Can you work these out from the model? Positions are in its coordinate system, mm. Face numbers are marked on the shaded views. A direction names the side the tool comes from. Coordinates: 2 decimals unless noted, no trailing zeros. Loops run counter-clockwise (first coordinate to the right, second up) from the corner with the lowest first, then second, coordinate; pieces in that order, holes last. Notation, with made-up numbers: (22.25, 46.5) -> (51.25, 46.5) arc R23 ccw to (51.25, 59.5) -> close; hole circle Ø10 at (34, 81.5). An arc over 180 degrees is marked (long way). Put each result on its own line as item: value. Start each with the question number.
Item 1: If we section it at A-A on x = -40.62: Please give me the cut outline in (y, z) (3 decimals), plus the area to 3 significant figures.
Item 2: For the marked faces 1, 2 and 3, which set-ups out of +Z, -Z, +X, -X, +Y, -Y let a thin tool reach every point of the face, with its end or its side?
Item 3: We'd pull the mould along X, two halves only. Please class the marked faces 4, 5, 6 and 7: pulls with the +X half, pulls with the -X half, needs draft (parallel to the pull), parting line crosses it, or undercut.
Item 4: If we section it at D-D on x = -27: Please give me the cut outline in (y, z).
Item 5: Will these pins go through, and if not, where does the flat tip stop? P1, Ø3, axis at x = -40.5, z = 4.5, coming from the +Y side; P2, Ø4, axis at x = -40.62, z = 20.685, coming from the -Y side; P3, Ø4, axis at y = 10.5, z = 16.5, coming from the -X side; P4, Ø3.5, axis at x = -15, z = 27.5, coming from the +Y side.
Item 6: Please list where these lines run through material, in increasing order: L1, parallel to X at y = 1.5, z = 23.38 (3 decimals); L2, parallel to Z at x = -14.5, y = 3.5; L3, parallel to X at y = 7.5, z = 2.5. Write a range as from..to.
Item 7: If we section it at B-B on y = 10: Please give me the cut outline in (x, z), plus the area to 3 significant figures.
Item 8: If we section it at C-C on z = 11: Please give me the cut outline in (x, y).
```python
from build123d import *

# Parameters (mm, degrees)
BOSS_EXTRUDE1_DEPTH = 3
BOSS_EXTRUDE2_START = 3
SKETCH1_3_W         = 52.27
SKETCH1_3_H         = 26.56
BOSS_EXTRUDE2_DEPTH = 8.6
BOSS_EXTRUDE3_START = 3
SKETCH1_4_R         = 1.25
SKETCH1_4_R_2       = 5
BOSS_EXTRUDE3_DEPTH = 3.4
CUT_EXTRUDE1_REACH  = 65.526
SKETCH2_W           = 18
SKETCH2_H           = 3.5
CUT_EXTRUDE2_REACH  = 65.627
SKETCH4_W           = 12
SKETCH4_H           = 6.2
SKETCH1_5_R         = 1.25
CUT_EXTRUDE3_DEPTH  = 64.410066236


with BuildPart() as part:
    # Sketch1 → Boss-Extrude1 (new body)
    with BuildSketch(Plane(origin=(0, 0, 0), x_dir=(1, 0, 0), z_dir=(0, 1, 0))):
        with BuildLine():
            Line((-0.75, 3.25), (-51.02, 3.25))
            ThreePointArc((-51.02, 3.25), (-53.848427125, 2.078427125), (-55.02, -0.75))
            Line((-55.02, -0.75), (-55.02, -25.31))
            ThreePointArc((-55.02, -25.31), (-53.848427125, -28.138427125), (-51.02, -29.31))
            Line((-51.02, -29.31), (-0.75, -29.31))
            ThreePointArc((-0.75, -29.31), (2.078427125, -28.138427125), (3.25, -25.31))
            Line((3.25, -25.31), (3.25, -0.75))
            ThreePointArc((3.25, -0.75), (2.078427125, 2.078427125), (-0.75, 3.25))
        make_face()
    extrude(amount=BOSS_EXTRUDE1_DEPTH)

    # Sketch1<3> → Boss-Extrude2 (add)
    with BuildSketch(Plane(origin=(0, 0, 0), x_dir=(1, 0, 0), z_dir=(0, 1, 0)).offset(BOSS_EXTRUDE2_START)):
        with BuildLine():
            ThreePointArc((3.25, -0.75), (2.078427125, 2.078427125), (-0.75, 3.25))
            Line((-0.75, 3.25), (-51.02, 3.25))
            ThreePointArc((-51.02, 3.25), (-53.848427125, 2.078427125), (-55.02, -0.75))
            Line((-55.02, -0.75), (-55.02, -25.31))
            ThreePointArc((-55.02, -25.31), (-53.848427125, -28.138427125), (-51.02, -29.31))
            Line((-51.02, -29.31), (-0.75, -29.31))
            ThreePointArc((-0.75, -29.31), (2.078427125, -28.138427125), (3.25, -25.31))
            Line((3.25, -25.31), (3.25, -0.75))
        make_face()
        with Locations((-25.885, -13.03)):
            Rectangle(SKETCH1_3_W, SKETCH1_3_H, mode=Mode.SUBTRACT)
    extrude(amount=BOSS_EXTRUDE2_DEPTH)

    # Sketch1<4> → Boss-Extrude3 (add)
    # profile 1 of 4: a face of its own
    with BuildSketch(Plane(origin=(0, 0, 0), x_dir=(1, 0, 0), z_dir=(0, 1, 0)).offset(BOSS_EXTRUDE3_START)):
        with BuildLine():
            Line((0, 0), (-6.949288811, 0))
            ThreePointArc((-6.949288811, 0), (-6.559292713, -6.566539242), (0, -7.063745122))
            Line((0, -7.063745122), (0, 0))
        make_face()
        with Locations(Location((-2.995, -3.06, 0), (0, 0, 270))):
            Circle(SKETCH1_4_R, mode=Mode.SUBTRACT)
    # profile 2 of 4: a face of its own
    with BuildSketch(Plane(origin=(0, 0, 0), x_dir=(1, 0, 0), z_dir=(0, 1, 0)).offset(BOSS_EXTRUDE3_START)):
        with Locations(Location((-40.62, -5.375, 0), (0, 0, 270))):
            Circle(SKETCH1_4_R_2)
        with Locations(Location((-40.62, -5.375, 0), (0, 0, 270))):
            Circle(SKETCH1_4_R, mode=Mode.SUBTRACT)
    # profile 3 of 4: a face of its own
    with BuildSketch(Plane(origin=(0, 0, 0), x_dir=(1, 0, 0), z_dir=(0, 1, 0)).offset(BOSS_EXTRUDE3_START)):
        with Locations(Location((-40.62, -20.685, 0), (0, 0, 270))):
            Circle(SKETCH1_4_R_2)
        with Locations(Location((-40.62, -20.685, 0), (0, 0, 270))):
            Circle(SKETCH1_4_R, mode=Mode.SUBTRACT)
    # profile 4 of 4: a face of its own
    with BuildSketch(Plane(origin=(0, 0, 0), x_dir=(1, 0, 0), z_dir=(0, 1, 0)).offset(BOSS_EXTRUDE3_START)):
        with BuildLine():
            Line((0, -26.06), (0, -19.376254878))
            ThreePointArc((0, -19.376254878), (-6.392636874, -19.711749235), (-7.216089907, -26.06))
            Line((-7.216089907, -26.06), (0, -26.06))
        make_face()
        with Locations(Location((-2.995, -23.38, 0), (0, 0, 270))):
            Circle(SKETCH1_4_R, mode=Mode.SUBTRACT)
    extrude(amount=BOSS_EXTRUDE3_DEPTH)

    # Sketch2 → Cut-Extrude1 (cut, up to next)
    with BuildSketch(Plane(origin=(0, 0, 26.31), x_dir=(-1, 0, 0), z_dir=(0, 0, -1)), mode=Mode.PRIVATE) as cut_extrude1_sk1:
        with Locations((12.45, 9.85)):
            Rectangle(SKETCH2_W, SKETCH2_H)
    cut_extrude1_tool1 = extrude(cut_extrude1_sk1.sketch, amount=-CUT_EXTRUDE1_REACH, mode=Mode.PRIVATE) & part.part
    add(cut_extrude1_tool1.solids().sort_by_distance((-12.45, 9.85, 26.31))[0], mode=Mode.SUBTRACT)

    # Sketch4 → Cut-Extrude2 (cut, up to next)
    with BuildSketch(Plane(origin=(-52.02, 0, 0), x_dir=(0, 0, -1), z_dir=(1, 0, 0)), mode=Mode.PRIVATE) as cut_extrude2_sk1:
        with Locations((-13.17934126, 8.5)):
            Rectangle(SKETCH4_W, SKETCH4_H)
    cut_extrude2_tool1 = extrude(cut_extrude2_sk1.sketch, amount=-CUT_EXTRUDE2_REACH, mode=Mode.PRIVATE) & part.part
    add(cut_extrude2_tool1.solids().sort_by_distance((-52.02, 8.5, 13.179341))[0], mode=Mode.SUBTRACT)

    # Sketch1<5> → Cut-Extrude3 (cut, through all)
    with BuildSketch(Plane(origin=(0, 0, 0), x_dir=(1, 0, 0), z_dir=(0, 1, 0))):
        with Locations(Location((-2.995, -23.38, 0), (0, 0, 270))):
            Circle(SKETCH1_5_R)
        with Locations(Location((-2.995, -3.06, 0), (0, 0, 270))):
            Circle(SKETCH1_5_R)
        with Locations(Location((-40.62, -5.375, 0), (0, 0, 270))):
            Circle(SKETCH1_5_R)
        with Locations(Location((-40.62, -20.685, 0), (0, 0, 270))):
            Circle(SKETCH1_5_R)
    extrude(amount=CUT_EXTRUDE3_DEPTH, mode=Mode.SUBTRACT)


solid = part.part
```
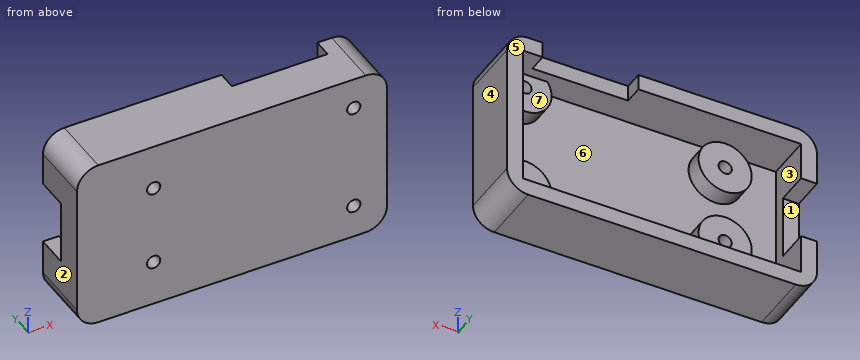
Solutions:
1. outline: (0, -3.25) -> (11.6, -3.25) -> (11.6, -0.25) -> (3, -0.25) -> (3, 0.375) -> (6.4, 0.375) -> (6.4, 4.125) -> (0, 4.125) -> close; (0, 6.625) -> (6.4, 6.625) -> (6.4, 10.375) -> (3, 10.375) -> (3, 15.685) -> (6.4, 15.685) -> (6.4, 19.435) -> (0, 19.435) -> close; (0, 21.935) -> (6.4, 21.935) -> (6.4, 25.685) -> (3, 25.685) -> (3, 26.31) -> (11.6, 26.31) -> (11.6, 29.31) -> (0, 29.31) -> close
1. area: 185 mm^2
2. face 1: -X, +Y
2. face 2: +Z, -Z, -X, +Y, -Y
2. face 3: +Y
3. face 4: pulls with the +X half
3. face 5: needs draft
3. face 6: undercut
3. face 7: undercut
4. outline: (0, -3.25) -> (11.6, -3.25) -> (11.6, -0.25) -> (3, -0.25) -> (3, 26.31) -> (11.6, 26.31) -> (11.6, 29.31) -> (0, 29.31) -> close
5. P1: y = 6.4
5. P2: y = 0
5. P3: x = 0.25
5. P4: y = 8.1
6. L1: -55.02..-4.245, -1.745..3.25
6. L2: -3.25..-0.25, 26.31..29.31
6. L3: -55.02..-52.02, 0.25..3.25
7. outline: (-55.02, 0.75) arc R4 ccw to (-51.02, -3.25) -> (-0.75, -3.25) arc R4 ccw to (3.25, 0.75) -> (3.25, 25.31) arc R4 ccw to (-0.75, 29.31) -> (-3.45, 29.31) -> (-3.45, 26.31) -> (0.25, 26.31) -> (0.25, -0.25) -> (-52.02, -0.25) -> (-52.02, 7.18) -> (-55.02, 7.18) -> close; (-55.02, 19.18) -> (-52.02, 19.18) -> (-52.02, 26.31) -> (-21.45, 26.31) -> (-21.45, 29.31) -> (-51.02, 29.31) arc R4 ccw to (-55.02, 25.31) -> close
7. area: 405 mm^2
8. outline: (-55.02, 0) -> (3.25, 0) -> (3.25, 11.6) -> (0.25, 11.6) -> (0.25, 3) -> (-52.02, 3) -> (-52.02, 5.4) -> (-55.02, 5.4) -> close
